Could you check a few things on this model? Use its own coordinates, in mm. A direction names the side the tool comes from. Round coordinates to 2 decimals unless told otherwise and drop trailing zeros. Write each loop counter-clockwise with the first axis right and the second up, starting at its lowest first coordinate (ties: lowest second). Pieces come first, ordered by that corner, then holes. Notation, with made-up numbers: M 76,58.25 L 106,58.25 A24 cw 106,70.25 Z; hole C 34.5,-0.75 d8. An arc over 180 degrees is marked long. One line per item, written item: value. Start each with the question number.
(1) I want a section at A-A on z = 10.5. Please give me the cut outline in (x, y), and give its area (3 significant figures).
(2) Which directions (+Z, -Z, +X, -X, +Y, -Y) give clear straight access to the entire face, cutting with the end or side of a thin tool? Please do faces 5 (the face through (-30.494, 24.286, 11.888)), 6 (the face through (-26, -24, 7)).
(3) If I drill on L1, parallel to Y at x = 24, z = 13.25; L2, parallel to Y at x = -24, z = 17.9; L3, parallel to Y at x = -24, z = 3, over which ranges is the centre line in solid material (lowest first)?
(4) I want a section at D-D on y = -24. Please give me the cut outline in (x, z), and give its area (3 significant figures).
(5) I'm going to push flat-ended pins straight in: pin 1 Ø6.5 at (x, y) = (24, 24) entering from +Z; pin 2 Ø1.5 at (y, z) = (22, 13.5) entering from -X; pin 3 Ø1.5 at (y, z) = (17.5, 9.5) entering from +X. Where does each tip first touch, or does it pass through?
(6) Thinking about a two-plate mould opening in Y: for faces 1 (the face through (34, -78, 2)), 2 (the face through (22, -25, 20)), 3 (the face through (-34, 33, 2)), 4 (the face through (19.209, -19.607, 11.888)), which applies, released by +Y, released by -Y, zero draft, split by the parting line, or undercut?
(7) I want a section at B-B on x = -24. Please give me the cut outline in (y, z).
(8) I want a section at C-C on y = 24. Please give me the cut outline in (x, z).
```python
from build123d import *

# Parameters (mm, degrees)
SKETCH1_R           = 6.5
BOSS_EXTRUDE1_DEPTH = 4
SKETCH1_5_R         = 6.5
SKETCH1_5_R_2       = 4
SKETCH1_5_R_3       = 2
BOSS_EXTRUDE2_DEPTH = 20
CUT_EXTRUDE1_START  = 20
SKETCH1_6_R         = 4
SKETCH1_6_R_2       = 2
CUT_EXTRUDE1_DEPTH  = 5


with BuildPart() as part:
    # Sketch1 → Boss-Extrude1 (new body)
    with BuildSketch(Plane.XY):
        with BuildLine():
            Line((-30, 35), (30, 35))
            ThreePointArc((30, 35), (33.535533906, 33.535533906), (35, 30))
            Line((35, 30), (35, -75))
            ThreePointArc((35, -75), (33.535533906, -78.535533906), (30, -80))
            Line((30, -80), (-30, -80))
            ThreePointArc((-30, -80), (-33.535533906, -78.535533906), (-35, -75))
            Line((-35, -75), (-35, 30))
            ThreePointArc((-35, 30), (-33.535533906, 33.535533906), (-30, 35))
        make_face()
        with Locations((24, -24)):
            Circle(SKETCH1_R, mode=Mode.SUBTRACT)
        with Locations((24, 24)):
            Circle(SKETCH1_R, mode=Mode.SUBTRACT)
        with Locations((-24, 24)):
            Circle(SKETCH1_R, mode=Mode.SUBTRACT)
        with Locations((-24, -24)):
            Circle(SKETCH1_R, mode=Mode.SUBTRACT)
    extrude(amount=BOSS_EXTRUDE1_DEPTH)

    # Sketch1_5 → Boss-Extrude2 (add)
    with BuildSketch(Plane.XY):
        with Locations((-24, -24)):
            Circle(SKETCH1_5_R)
        with Locations((-24, -24)):
            Circle(SKETCH1_5_R_2, mode=Mode.SUBTRACT)
        with Locations((-24, -24)):
            Circle(SKETCH1_5_R_2)
        with Locations((-24, -24)):
            Circle(SKETCH1_5_R_3, mode=Mode.SUBTRACT)
        with Locations((24, -24)):
            Circle(SKETCH1_5_R)
        with Locations((24, -24)):
            Circle(SKETCH1_5_R_2, mode=Mode.SUBTRACT)
        with Locations((24, -24)):
            Circle(SKETCH1_5_R_2)
        with Locations((24, -24)):
            Circle(SKETCH1_5_R_3, mode=Mode.SUBTRACT)
        with Locations((24, 24)):
            Circle(SKETCH1_5_R)
        with Locations((24, 24)):
            Circle(SKETCH1_5_R_2, mode=Mode.SUBTRACT)
        with Locations((24, 24)):
            Circle(SKETCH1_5_R_2)
        with Locations((24, 24)):
            Circle(SKETCH1_5_R_3, mode=Mode.SUBTRACT)
        with Locations((-24, 24)):
            Circle(SKETCH1_5_R)
        with Locations((-24, 24)):
            Circle(SKETCH1_5_R_2, mode=Mode.SUBTRACT)
        with Locations((-24, 24)):
            Circle(SKETCH1_5_R_2)
        with Locations((-24, 24)):
            Circle(SKETCH1_5_R_3, mode=Mode.SUBTRACT)
    extrude(amount=BOSS_EXTRUDE2_DEPTH)

    # Sketch1_6 → Cut-Extrude1 (cut)
    with BuildSketch(Plane.XY.offset(CUT_EXTRUDE1_START)):
        with Locations((24, 24)):
            Circle(SKETCH1_6_R)
        with Locations((24, 24)):
            Circle(SKETCH1_6_R_2, mode=Mode.SUBTRACT)
        with Locations((-24, 24)):
            Circle(SKETCH1_6_R)
        with Locations((-24, 24)):
            Circle(SKETCH1_6_R_2, mode=Mode.SUBTRACT)
        with Locations((-24, -24)):
            Circle(SKETCH1_6_R)
        with Locations((-24, -24)):
            Circle(SKETCH1_6_R_2, mode=Mode.SUBTRACT)
        with Locations((24, -24)):
            Circle(SKETCH1_6_R_2)
    extrude(amount=-CUT_EXTRUDE1_DEPTH, mode=Mode.SUBTRACT)


solid = part.part
```
Found:
1. outline: C -24,-24 d13; C -24,24 d13; C 24,-24 d13; C 24,24 d13; hole C -24,-24 d4; hole C -24,24 d4; hole C 24,-24 d4; hole C 24,24 d4
1. area: 481 mm²
2. face 5: +Z
2. face 6: +Z, -Z
3. L1: y = -30.5 to -26, -22 to -17.5, 17.5 to 22, 26 to 30.5
3. L2: y = -30.5 to -28, -20 to -17.5, 17.5 to 20, 28 to 30.5
3. L3: y = -80 to -26, -22 to 22, 26 to 35
4. outline: M -35,0 L -26,0 L -26,15 L -28,15 L -28,20 L -30.5,20 L -30.5,4 L -35,4 Z; M -22,0 L 22,0 L 22,20 L 17.5,20 L 17.5,4 L -17.5,4 L -17.5,20 L -20,20 L -20,15 L -22,15 Z; M 26,0 L 35,0 L 35,4 L 30.5,4 L 30.5,20 L 26,20 Z
4. area: 516 mm²
5. pin 1: stops at z = 15
5. pin 2: stops at x = -30.38
5. pin 3: stops at x = 27.03
6. face 1: released by -Y
6. face 2: zero draft
6. face 3: released by +Y
6. face 4: undercut
7. outline: M -80,0 L -26,0 L -26,15 L -28,15 L -28,20 L -30.5,20 L -30.5,4 L -80,4 Z; M -22,0 L 22,0 L 22,15 L 20,15 L 20,20 L 17.5,20 L 17.5,4 L -17.5,4 L -17.5,20 L -20,20 L -20,15 L -22,15 Z; M 26,0 L 35,0 L 35,4 L 30.5,4 L 30.5,20 L 28,20 L 28,15 L 26,15 Z
8. outline: M -35,0 L -26,0 L -26,15 L -28,15 L -28,20 L -30.5,20 L -30.5,4 L -35,4 Z; M -22,0 L 22,0 L 22,15 L 20,15 L 20,20 L 17.5,20 L 17.5,4 L -17.5,4 L -17.5,20 L -20,20 L -20,15 L -22,15 Z; M 26,0 L 35,0 L 35,4 L 30.5,4 L 30.5,20 L 28,20 L 28,15 L 26,15 Z
